Can you work these out from the model? Positions are in its coordinate system, mm. A direction names the side the tool comes from. Give positions to 0.01 mm unless a question says otherwise; leave off trailing zeros. Write each loop counter-clockwise with the first axis right and the second up, starting at its lowest first coordinate (ties: lowest second). Pieces come first, ordered by that corner, then holes.
```python
from build123d import *

# Parameters (mm, degrees)
F0_W     = 126
F0_H     = 88
F0_R     = 2.5
F1_DEPTH = 3
F2_DEPTH = 35
F3_START = 33
F3_DEPTH = 2
F4_SIZE  = 1


with BuildPart() as f1:
    # F0 (on Top) → F1 (new body)
    with BuildSketch(Plane.XY):
        with Locations((0, 44)):
            Rectangle(F0_W, F0_H)
        with Locations((-51.5, 80.5)):
            Circle(F0_R, mode=Mode.SUBTRACT)
        with Locations((51.5, 80.5)):
            Circle(F0_R, mode=Mode.SUBTRACT)
        Polygon((65, -90), (65, 0), (63, 0), (63, -88), (-63, -88), (-63, 0), (-65, 0), (-65, -90), align=None)
        Polygon((65, 0), (65, 90), (-65, 90), (-65, 0), (-63, 0), (-63, 88), (63, 88), (63, 0), align=None)
        with Locations((0, -44)):
            Rectangle(F0_W, F0_H)
        with Locations((-51.5, -80.5)):
            Circle(F0_R, mode=Mode.SUBTRACT)
        with Locations((51.5, -80.5)):
            Circle(F0_R, mode=Mode.SUBTRACT)
    extrude(amount=-F1_DEPTH)

    # F0 (on Top) → F2 (join)
    with BuildSketch(Plane.XY):
        Polygon((65, 0), (65, 90), (-65, 90), (-65, 0), (-63, 0), (-63, 88), (63, 88), (63, 0), align=None)
    extrude(amount=F2_DEPTH)

    # F0 (on Top) → F3 (join)
    with BuildSketch(Plane.XY.offset(F3_START)):
        with Locations((0, 44)):
            Rectangle(F0_W, F0_H)
        with Locations((-51.5, 80.5)):
            Circle(F0_R, mode=Mode.SUBTRACT)
        with Locations((51.5, 80.5)):
            Circle(F0_R, mode=Mode.SUBTRACT)
        Polygon((65, 0), (65, 90), (-65, 90), (-65, 0), (-63, 0), (-63, 88), (63, 88), (63, 0), align=None)
        with Locations((-51.5, 80.5)):
            Circle(F0_R)
        with Locations((51.5, 80.5)):
            Circle(F0_R)
    extrude(amount=F3_DEPTH)

    # F4
    f4_edges = [f1.edges().sort_by_distance(p)[0] for p in [
        (65, 45, 35),
        (0, 90, 35),
        (-65, 45, 35),
        (0, 0, 35),
        (-65, 0, -3),
        (-65, -90, -1.5),
        (-65, -45, 0),
        (-65, 0, 17.5),
        (-65, 90, 16),
        (65, 90, 16),
        (0, 90, -3),
        (65, -45, 0),
        (65, -90, -1.5),
        (65, 0, -3),
        (65, 0, 17.5),
        (-54, 80.5, -3),
        (49, 80.5, -3),
        (0, -90, -3),
        (-54, -80.5, -3),
        (49, -80.5, -3),
    ]]
    chamfer(f4_edges, length=F4_SIZE)


solid = f1.part
```
1) Please list where these lines run through material, in increasing order: L1, parallel to Y at x = 51.5, z = -0.65; L2, parallel to Z at x = 57, y = 4; L3, parallel to X at y = 51.5, z = 28.
Values follow:
L1: y = -90 to -83, -78 to 78, 83 to 90
L2: z = -3 to 0, 33 to 35
L3: x = -65 to -63, 63 to 65
2) Suppose I cut it at D-D on x = 16. Write out the boundary of the cut face in (y, z).
Values follow:
outline: (-90, -2) - (-89, -3) - (89, -3) - (90, -2) - (90, 34) - (89, 35) - (1, 35) - (0, 34) - (0, 33) - (88, 33) - (88, 0) - (-90, 0) - close
3) Suppose I cut it at C-C on y = -80.5. Write out the boundary of the cut face in (x, z), plus the area to 3 significant figures.
Values follow:
outline: (-65, -2) - (-64, -3) - (-55, -3) - (-54, -2) - (-54, 0) - (-64, 0) - (-65, -1) - close; (-49, -2) - (-48, -3) - (48, -3) - (49, -2) - (49, 0) - (-49, 0) - close; (54, -2) - (55, -3) - (64, -3) - (65, -2) - (65, -1) - (64, 0) - (54, 0) - close
area: 356 mm2
4) Suppose I cut it at A-A on x = -51.5. Write out the boundary of the cut face in (y, z), plus the area to 3 significant figures.
Values follow:
outline: (-90, -2) - (-89, -3) - (-84, -3) - (-83, -2) - (-83, 0) - (-90, 0) - close; (-78, -2) - (-77, -3) - (77, -3) - (78, -2) - (78, 0) - (-78, 0) - close; (0, 33) - (88, 33) - (88, 0) - (83, 0) - (83, -2) - (84, -3) - (89, -3) - (90, -2) - (90, 34) - (89, 35) - (1, 35) - (0, 34) - close
area: 752 mm2
5) If we mould it in two halves opening along X, with no side actions, what happens to faces 1 (the face through (65, 58, 16)), 2 (the face through (53.81, -81.46, -0.99)), 3 (the face through (-1, 1, -3))? For each: +X half, -X half, draft (parallel to the pull), parting line (faces both ways), or undercut.
Values follow:
face 1: +X half
face 2: undercut
face 3: draft
6) Suppose I cut it at B-B on y = 80.5. Write out the boundary of the cut face in (x, z), plus the area to 3 significant figures.
Values follow:
outline: (-65, -2) - (-64, -3) - (-55, -3) - (-54, -2) - (-54, 0) - (-63, 0) - (-63, 33) - (63, 33) - (63, 0) - (54, 0) - (54, -2) - (55, -3) - (64, -3) - (65, -2) - (65, 34) - (64, 35) - (-64, 35) - (-65, 34) - close; (-49, -2) - (-48, -3) - (48, -3) - (49, -2) - (49, 0) - (-49, 0) - close
area: 748 mm2
7) For pin 1 Ø6 at (x, y) = (-51.5, -80.5) entering from -Z; pin 2 Ø6.5 at (x, y) = (51.5, 80.5) entering from -Z; pin 3 Ø4.5 at (x, y) = (51.5, -80.5) entering from -Z; pin 4 Ø3 at (x, y) = (28.5, -61.5) entering from +Z, each with a flat end and sliding along its axis, tell me the tip position at first contact or that it passes through.
Values follow:
pin 1: stops at z = -2.5
pin 2: stops at z = -2.75
pin 3: passes through
pin 4: stops at z = 0
8) For faces 4 (the face through (63, 45, 16)), 5 (the face through (-49.19, 79.54, -0.99)), 6 (the face through (-0.3, 0, 33.3)), which set-ups out of +Z, -Z, +X, -X, +Y, -Y let a thin tool reach every point of the face, with its end or its side?
Values follow:
face 4: -Y
face 5: -Z
face 6: +Z, +X, -X, -Y
